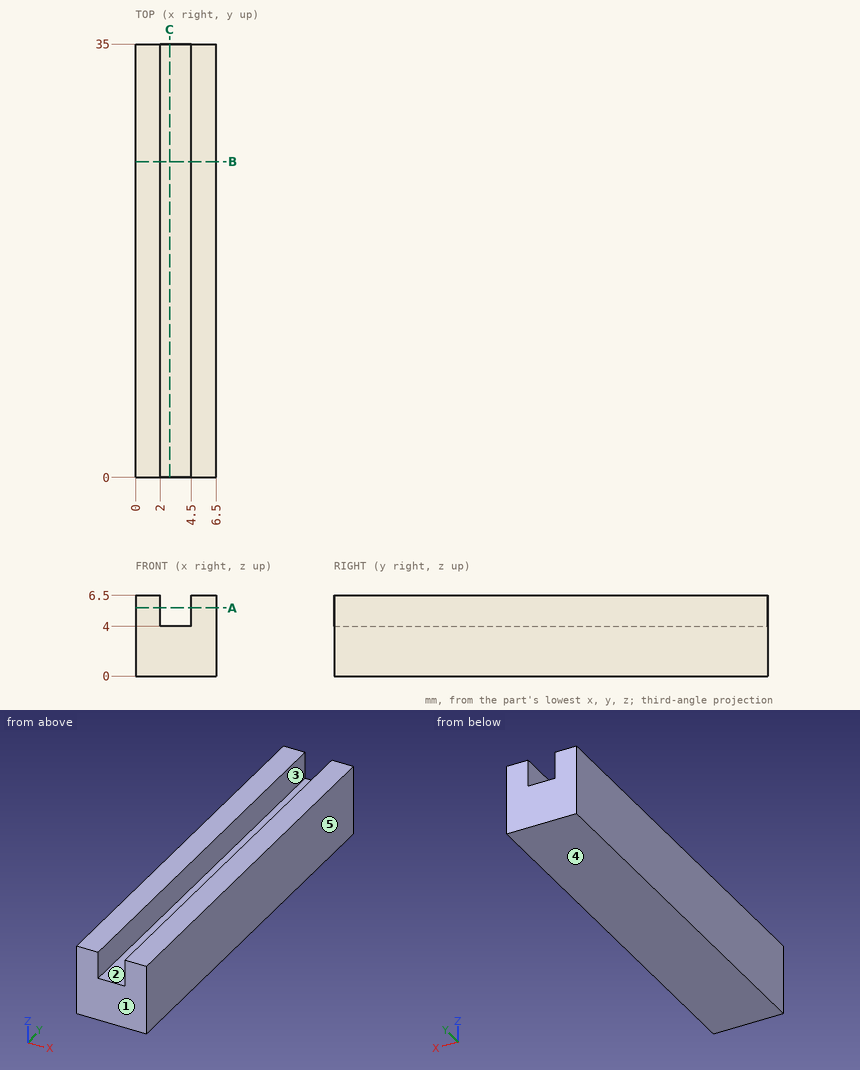
Drawing for the job (mm, zero at the part's lowest x, y, z). A direction names the side the tool comes from. Coordinates: 2 decimals unless noted, no trailing zeros. Order: outer loops, then holes, each group sorted by start corner. A loop starts at its lowest first (then second) coordinate and runs counter-clockwise, first axis right, second up.
Item 1: Drill centre lines: L1, parallel to X at y = 6, z = 5.25; L2, parallel to Z at x = 3.75, y = 21. Where is each one in solid material? Low to high.
Check sheet entries:
L1: x = 0 to 2, 4.5 to 6.5
L2: z = 0 to 4
Item 2: Pin check, flat tip, straight feed: pin 1 Ø2 at (x, z) = (4, 2.5) entering from -Y. Stop position of the tip, or through.
Check sheet entries:
pin 1: stops at y = 0
Item 3: Band-saw the part on C-C on x = 2.75. List the corners of the cut face in (y, z), plus the area to 3 significant figures.
Check sheet entries:
outline: (0, 0) - (35, 0) - (35, 4) - (0, 4) - close
area: 140 mm2
Item 4: Two-plate mould, pull along X, no slides. Class the marked faces 3, 4 and 5: +X half, -X half, draft (parallel to the pull), parting line (faces both ways), or undercut.
Check sheet entries:
face 3: undercut
face 4: draft
face 5: +X half
Item 5: 3-axis set-ups, long thin cutter, end or side, ignore diameter. For the marked faces 1 and 2: which of +Z, -Z, +X, -X, +Y, -Y reach the whole face in a straight line?
Check sheet entries:
face 1: +Z, -Z, +X, -X, -Y
face 2: +Z, +Y, -Y
Item 6: Band-saw the part on A-A on z = 5.5. List the corners of the cut face in (x, y), plus the area to 3 significant figures.
Check sheet entries:
outline: (0, 0) - (2, 0) - (2, 35) - (0, 35) - close; (4.5, 0) - (6.5, 0) - (6.5, 35) - (4.5, 35) - close
area: 140 mm2
Item 7: Band-saw the part on B-B on y = 25.5. List the corners of the cut face in (x, z), plus the area to 3 significant figures.
Check sheet entries:
outline: (0, 0) - (6.5, 0) - (6.5, 6.5) - (4.5, 6.5) - (4.5, 4) - (2, 4) - (2, 6.5) - (0, 6.5) - close
area: 36.0 mm2
